```python
from build123d import *

# Parameters (mm, degrees)
PAD_DEPTH          = 19.9
SKETCH001_R        = 2.55
POCKET_DEPTH       = 550.545928
POLARPATTERN_COUNT = 6


with BuildPart() as part:
    # Sketch → Pad (new body)
    with BuildSketch(Plane.XY):
        Polygon((0, 100), (-86.60254, 50), (-86.60254, -50), (0, -100), (86.60254, -50), (86.60254, 50), align=None)
        Polygon((-13.95, 0), (-6.975, -12.081054), (6.975, -12.081054), (13.95, 0), (6.975, 12.081054), (-6.975, 12.081054), align=None, mode=Mode.SUBTRACT)
    extrude(amount=PAD_DEPTH)

    # Sketch001 (on Face14 of Pad) → Pocket (cut, through all)
    with BuildSketch(Plane.XY.offset(19.9)):
        with Locations((80.1, 25)):
            Circle(SKETCH001_R)
        with Locations((80.1, -25)):
            Circle(SKETCH001_R)
        with Locations((80.1, 0)):
            Circle(SKETCH001_R)
    pocket = extrude(amount=-POCKET_DEPTH, mode=Mode.SUBTRACT)

    # PolarPattern: Pocket ×6 about axis
    polarpattern_axis = Axis((0, 0, 19.9), (0, 0, 1))
    for i in range(1, POLARPATTERN_COUNT):
        add(pocket.rotate(polarpattern_axis, i * 360 / POLARPATTERN_COUNT), mode=Mode.SUBTRACT)


solid = part.part
```
Here's how the part is built. I have some questions about the finished solid (model axes, mm). A direction names the side the tool comes from. Give positions to 0.01 mm unless a question says otherwise; leave off trailing zeros. Write each loop counter-clockwise with the first axis right and the second up, starting at its lowest first coordinate (ties: lowest second). Pieces come first, ordered by that corner, then holes. Notation, with made-up numbers: (51, 19) -> (85, 19) arc R27 ccw to (85, 35) -> close; hole circle Ø9 at (24.25, 57.5). An arc over 180 degrees is marked (long way). Use one line per item in the form item = value.
1) If I drill on L1, parallel to Y at x = -60, z = 18.75; L2, parallel to Y at x = -40.05, z = 4.25; L3, parallel to Y at x = 0, z = 14.5, over which ranges is the centre line in solid material (lowest first)? Write a range as [from, to].
Verdict:
L1 = [-65.36, -58.77], [-54.97, 54.97], [58.77, 65.36]
L2 = [-76.88, -71.92], [-66.82, 66.82], [71.92, 76.88]
L3 = [-100, -12.08], [12.08, 100]
2) Suppose I cut it at C-C (z = 17.75). Give the number of separate pieces and of enclosed holes in the cut face, and give its area (3 significant figures).
Verdict:
separate_pieces = 1
enclosed_holes = 19
area = 25,100 mm2
3) Suppose I cut it at A-A (y = 25). Please give me the cut outline in (x, z).
Verdict:
outline = (-86.6, 0) -> (-82.65, 0) -> (-82.65, 19.9) -> (-86.6, 19.9) -> close; (-77.55, 0) -> (77.55, 0) -> (77.55, 19.9) -> (-77.55, 19.9) -> close; (82.65, 0) -> (86.6, 0) -> (86.6, 19.9) -> (82.65, 19.9) -> close
4) I'm going to push flat-ended pins straight in: pin 1 (10 mm diameter, centred on x = 37.5, z = 16.5, fed in from +Y); pin 2 (11 mm diameter, centred on x = 1, z = 8.5, fed in from -Y); pin 3 (6 mm diameter, centred on x = -32.5, y = -26, fed in from -Z); pin 4 (4 mm diameter, centred on y = -66.5, z = 10.5, fed in from -X). Where does each tip first touch, or does it pass through?
Verdict:
pin_1 = 81.24
pin_2 = -100
pin_3 = 0
pin_4 = -61.49
5) Suppose I cut it at D-D (y = -5). Please give me the cut outline in (x, z).
Verdict:
outline = (-86.6, 0) -> (-11.06, 0) -> (-11.06, 19.9) -> (-86.6, 19.9) -> close; (11.06, 0) -> (86.6, 0) -> (86.6, 19.9) -> (11.06, 19.9) -> close
6) Suppose I cut it at B-B (x = -80.1). Please give me the cut outline in (y, z).
Verdict:
outline = (-53.75, 0) -> (-27.55, 0) -> (-27.55, 19.9) -> (-53.75, 19.9) -> close; (-22.45, 0) -> (-2.55, 0) -> (-2.55, 19.9) -> (-22.45, 19.9) -> close; (2.55, 0) -> (22.45, 0) -> (22.45, 19.9) -> (2.55, 19.9) -> close; (27.55, 0) -> (53.75, 0) -> (53.75, 19.9) -> (27.55, 19.9) -> close
7) We'd pull the mould along X, two halves only. Please class faces 1 (the face through (-86.603, 1, 10)), 2 (the face through (10.51, 5.96, 9.81)), 3 (the face through (0, -12.081, 10)), 4 (the face through (43.91, 74.65, 9.81)): +X half, -X half, draft (parallel to the pull), parting line (faces both ways), or undercut.
Verdict:
face_1 = -X half
face_2 = undercut
face_3 = undercut
face_4 = +X half
8) On a 3-axis mill with a long thin cutter (end or side, diameter ignored), from which of +Z, -Z, +X, -X, +Y, -Y can I reach the whole of each face in a straight line? I mean faces 5 (the face through (0, 12.081, 10)), 6 (the face through (86.603, -1, 10)). Say none if no direction works.
Verdict:
face_5 = +Z, -Z
face_6 = +Z, -Z, +X, +Y, -Y
